```python
from build123d import *

# Parameters (mm, degrees)
F0_W      = 104
F0_H      = 104
F1_DEPTH  = 2
F2_W      = 2
F2_H      = 104
F3_DEPTH  = 25
F4_W      = 2
F4_H      = 104
F5_DEPTH  = 25
F6_R      = 0.99999
F7_R      = 0.99999
F9_D      = 4
F11_D     = 4
F13_D     = 4
F15_DEPTH = 500
F16_DEPTH = 505


# Not quite as in the source:
# - a fillet or chamfer is up to 0.001 mm smaller than in the source, because OpenCascade refuses the exact size


with BuildPart() as f1:
    # F0 (on Top) → F1 (new body)
    with BuildSketch(Plane.XY):
        Rectangle(F0_W, F0_H)
    extrude(amount=F1_DEPTH)

    # F2 (on face) → F3 (join)
    with BuildSketch(Plane.XY.offset(2)):
        with Locations((-51, 0)):
            Rectangle(F2_W, F2_H)
    extrude(amount=F3_DEPTH)

    # F4 (on face) → F5 (join)
    with BuildSketch(Plane.XY.offset(2)):
        with Locations((51, 0)):
            Rectangle(F4_W, F4_H)
    extrude(amount=F5_DEPTH)

    # F6 (radius 1 in the source; OpenCascade refuses exactly that, so slightly less here)
    f6_edges = [f1.edges().sort_by_distance(p)[0] for p in [
        (52, 0, 27),
        (51, 52, 27),
        (50, 0, 27),
        (51, -52, 27),
    ]]
    fillet(f6_edges, radius=F6_R)

    # F7 (radius 1 in the source; OpenCascade refuses exactly that, so slightly less here)
    f7_edges = [f1.edges().sort_by_distance(p)[0] for p in [
        (-51, 52, 27),
        (-52, 0, 27),
        (-51, -52, 27),
        (-50, 0, 27),
    ]]
    fillet(f7_edges, radius=F7_R)

    # F9 (through all)
    with Locations(Plane.YZ.offset(52)):
        with Locations((-33, 17)):
            Hole(F9_D / 2)

    # F11 (through all)
    with Locations(Plane.YZ.offset(52)):
        with Locations((1, 17)):
            Hole(F11_D / 2)

    # F13 (through all)
    with Locations(Plane.YZ.offset(52)):
        with Locations((35, 17)):
            Hole(F13_D / 2)

    # F14 (on Front) → F15 (cut)
    with BuildSketch(Plane.XZ):
        Polygon((74.380248785, 39.0327088535), (-49.979981035, 2.7150458191), (-49.979981035, 0), (-49.979981035, -1.495702425), (74.380248785, -1.495702425), align=None)
    extrude(amount=F15_DEPTH, mode=Mode.SUBTRACT)

    # F14 (on Front) → F16 (cut)
    with BuildSketch(Plane.XZ):
        Polygon((74.380248785, 39.0327088535), (-49.979981035, 2.7150458191), (-49.979981035, 0), (-49.979981035, -1.495702425), (74.380248785, -1.495702425), align=None)
    extrude(amount=-F16_DEPTH, mode=Mode.SUBTRACT)


solid = f1.part
```
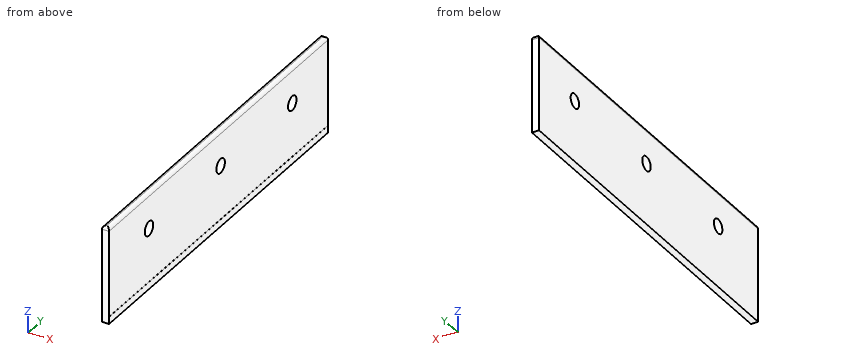
The listing builds one solid part. Answer for the finished solid, in the listing's coordinates (mm). Round coordinates to 2 decimals unless told otherwise and drop trailing zeros. Write each loop counter-clockwise with the first axis right and the second up, starting at its lowest first coordinate (ties: lowest second). Pieces come first, ordered by that corner, then holes. Notation, with made-up numbers: (86.5, 7) -> (111.5, 7) arc R16 ccw to (111.5, 17) -> close; hole circle Ø4 at (59.25, 71.5). An arc over 180 degrees is marked (long way). Answer as a JSON object with one key per item and string values. Group by question number.
Q1. Section B-B (z = 17) is taken. Write down the section's boundary in (x, y), plus the area to 3 significant figures.
Q2. Section C-C (x = -50.55) is taken. Write down the section's boundary in (y, z), plus the area to 3 significant figures.
Q3. Each of these flat-tipped pins is pushed along its axis until it touches: pin 1 Ø5 at (y, z) = (1, 17) entering from +X; pin 2 Ø3.5 at (y, z) = (-33, 17) entering from -X. Where does it stop, or does it pass through?
Q4. Straight lines are drawn through the part: line 1 along Z through (x, y) = (-50.8, 1); line 2 along X through (y, z) = (-8, 8.75); line 3 along Z through (x, y) = (-50.6, 35). For each, find the intervals that lie inside material, in ascending order.
Check values:
{
 "1": {"outline": "(-52, -52) -> (-50, -52) -> (-50, -35) -> (-52, -35) -> close; (-52, -31) -> (-50, -31) -> (-50, -1) -> (-52, -1) -> close; (-52, 3) -> (-50, 3) -> (-50, 33) -> (-52, 33) -> close; (-52, 37) -> (-50, 37) -> (-50, 52) -> (-52, 52) -> close", "area": "184 mm^2"},
 "2": {"outline": "(-52, 0) -> (52, 0) -> (52, 26) arc R1 ccw to (51.45, 26.89) -> (-51.45, 26.89) arc R1 ccw to (-52, 26) -> close; hole circle Ø4 at (-33, 17); hole circle Ø4 at (1, 17); hole circle Ø4 at (35, 17)", "area": "2,760 mm^2"},
 "3": {"pin 1": "x = -50", "pin 2": "through"},
 "4": {"line 1": "0 to 15, 19 to 26.98", "line 2": "-52 to -50", "line 3": "0 to 15, 19 to 26.92"}
}
